CAD build for the part. Positions are in the model's coordinates, mm. A direction names the side the tool comes from. Round coordinates to 2 decimals unless told otherwise and drop trailing zeros. Loops run counter-clockwise (first coordinate to the right, second up) from the corner with the lowest first, then second, coordinate; pieces in that order, holes last. Notation, with made-up numbers: (-12, 79) - (-7, 79) arc R27 ccw to (-7, 113) - close; hole circle Ø2 at (-21, 79.25). An arc over 180 degrees is marked (long way). One line per question, with ' | ' between items.
```python
from build123d import *

# Parameters (mm, degrees)
BOSS_EXTRUDE1_START = -21.2
SKETCH1_R           = 4
BOSS_EXTRUDE1_DEPTH = 50
SKETCH2_R           = 7
BOSS_EXTRUDE2_DEPTH = 4.4
CUT_EXTRUDE1_DEPTH  = 2.6
SKETCH5_R           = 2.886751346
CUT_EXTRUDE2_DEPTH  = 1
CUT_EXTRUDE2_DRAFT  = -45
CHAMFER1_SIZE       = 0.8


with BuildPart() as part:
    # Sketch1 → Boss-Extrude1 (new body)
    with BuildSketch(Plane.XY.offset(BOSS_EXTRUDE1_START)):
        with Locations((-20, 0)):
            Circle(SKETCH1_R)
    extrude(amount=-BOSS_EXTRUDE1_DEPTH)

    # Sketch2 → Boss-Extrude2 (add)
    with BuildSketch(Plane.XY.offset(-21.2)):
        with Locations((-20, 0)):
            Circle(SKETCH2_R)
    extrude(amount=BOSS_EXTRUDE2_DEPTH)

    # Sketch3 → Cut-Revolve1 (revolve, cut)
    with BuildSketch(Plane(origin=(-20, 0, 0), x_dir=(0, 0, -1), z_dir=(1, 0, 0))):
        with BuildLine():
            Line((16.8, 4), (15.8, 4))
            Line((15.8, 4), (15.8, 8))
            Line((15.8, 8), (20.9, 8))
            Line((20.9, 8), (20.9, 7))
            ThreePointArc((20.9, 7), (18.312578573, 6.23447595), (16.8, 4))
        make_face()
    revolve(axis=Axis((-20, 0, -71.2), (0, 0, 1)), mode=Mode.SUBTRACT)

    # Sketch4 → Cut-Extrude1 (cut)
    with BuildSketch(Plane.XY.offset(-16.8)):
        Polygon((-20, 2.886751346), (-22.5, 1.443375673), (-22.5, -1.443375673), (-20, -2.886751346), (-17.5, -1.443375673), (-17.5, 1.443375673), align=None)
    extrude(amount=-CUT_EXTRUDE1_DEPTH, mode=Mode.SUBTRACT)


with BuildPart() as cut_extrude2_tool:
    # Sketch5 → Cut-Extrude2 (with draft: the straight prism first)
    with BuildSketch(Plane.XY.offset(-16.8)):
        with Locations((-20, 0)):
            Circle(SKETCH5_R)
    extrude(amount=-CUT_EXTRUDE2_DEPTH)
    # Cut-Extrude2: the draft: its side faces are tilted about the plane it starts from
    cut_extrude2_sides = [cut_extrude2_tool.faces().sort_by_distance(p)[0] for p in [
        (-22.886751346, 0, -17.3),
    ]]
    draft(cut_extrude2_sides, Plane.XY.offset(-16.8), CUT_EXTRUDE2_DRAFT)


with BuildPart() as part_1:
    add(part.part)

    # Cut-Extrude2: cut by cut_extrude2_tool
    add(cut_extrude2_tool.part, mode=Mode.SUBTRACT)

    # Chamfer1
    chamfer1_edges = [part_1.edges().sort_by_distance(p)[0] for p in [
        (-24, 0, -71.2),
    ]]
    chamfer(chamfer1_edges, length=CHAMFER1_SIZE)


solid = part_1.part
```
(1) Two-plate mould, pull along X, no slides. Class faces 4 (the face through (-20, 0, -71.2)), 5 (the face through (-21.37, -2.32, -16.99)), 6 (the face through (-27, 0, -21)): released by +X, released by -X, zero draft, split by the parting line, or undercut.
Results found:
face 4: zero draft | face 5: undercut | face 6: split by the parting line
(2) Tool access for faces 1 (the face through (-19, -3, -16.8)), 2 (the face through (-18.63, 2.32, -16.99)), 3 (the face through (-23.2, -2.4, -45.5)): list every direction of +Z, -Z, +X, -X, +Y, -Y with a clear straight run to the whole face (end or side of a thin tool).
Results found:
face 1: +Z, +X, -X, +Y, -Y | face 2: +Z | face 3: -Z
(3) Probe L1, parallel to Z at x = -19.75, y = -1.5; L2, parallel to X at y = -0.5, z = -26.5; L3, parallel to Z at x = -20.25, y = -6. List the from-to ranges inside material, lowest first.
Results found:
L1: z = -71.2 to -19.4 | L2: x = -23.97 to -16.03 | L3: z = -21.2 to -18.03
(4) Drop flat-ended pins along their axis: P1, Ø2.5, axis at x = -19, y = -1, coming from the +Z side; P2, Ø3, axis at y = 0.5, z = -18.5, coming from the +X side; P3, Ø8, axis at x = -17.5, z = -42, coming from the +Y side. Give the stop position or say it passes through.
Results found:
P1: stops at z = -17.02 | P2: stops at x = -13.06 | P3: stops at y = 4
(5) Cut at A-A, the plane z = -48.5. Write the cut outline in (x, y), then the cut area to 3 significant figures.
Results found:
outline: circle Ø8 at (-20, 0) | area: 50.3 mm²
